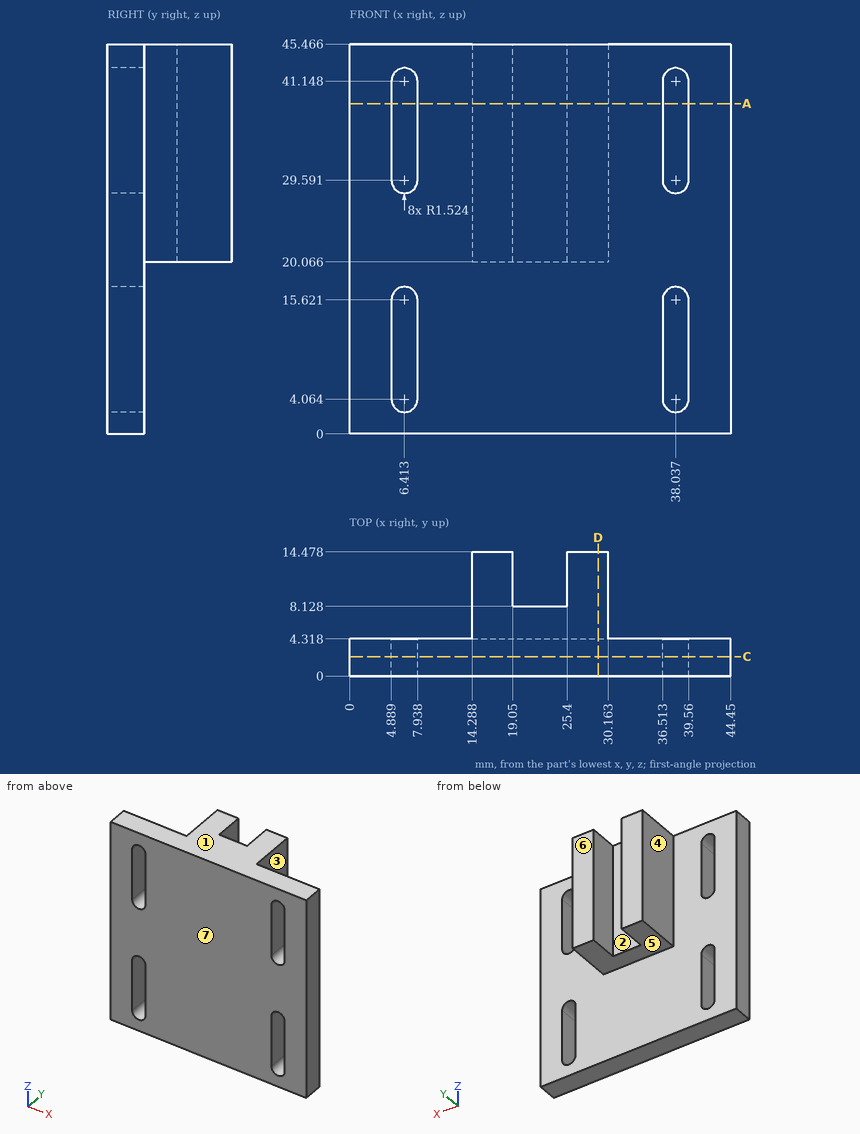
Source: three-view drawing plus pictorial views. Frame: mm from the lowest corner of the part. A direction names the side the tool comes from. Coordinates: 2 decimals unless noted, no trailing zeros. Order: outer loops, then holes, each group sorted by start corner. A loop starts at its lowest first (then second) coordinate and runs counter-clockwise, first axis right, second up. Notation, with made-up numbers: M -12.5,-32.5 L 17.5,-32.5 A10 ccw 17.5,-18.5 Z; hole C -11.5,76 d11. An arc over 180 degrees is marked long. One line per question, with ' | ' between items. Start each with the question number.
Item 1: Set-up query: the marked faces 1, 2, 3 and 4. Return all of +Z, -Z, +X, -X, +Y, -Y with unobstructed straight access to the full face (end or side cutting, diameter ignored); none if empty.
Item 2: Draft query along Y for the marked faces 5, 6 and 7. Return one class per face: released by +Y, released by -Y, zero draft, split by the parting line, or undercut.
Item 3: Ray query, probe 1 along X at (y, z) = (2.5, 13.5); probe 2 along X at (y, z) = (10.5, 38.5); probe 3 along Z at (x, y) = (7, 1) (1 decimal). Return the intervals inside material, ascending. Write a range as [from, to].
Item 4: Cut plane C-C, the plane y = 2.25. Count the separate pieces of the cut face and the enclosed holes in it, then the cut area to 3 significant figures.
Item 5: Pin query (flat end, axial travel): pin 1 Ø3 at (y, z) = (11, 32.5) entering from -X; pin 2 Ø5 at (x, y) = (38.5, 7) entering from +Z; pin 3 Ø5 at (x, y) = (21, 7.5) entering from -Z; pin 4 Ø10 at (x, z) = (5, 39) entering from +Y. Return the tip coordinate at first contact, or that it passes through.
Item 6: Cut plane A-A, the plane z = 38.5. Return the cut outline in (x, y).
Item 7: Cut plane D-D, the plane x = 29. Return the cut outline in (y, z) (1 decimal).
A:
1) face 1: +Z, +X, -X, +Y, -Y | face 2: +Z, -Z, +Y | face 3: +Z, -Z, +X, +Y | face 4: +Z, -Z, -X, +Y
2) face 5: zero draft | face 6: released by +Y | face 7: released by -Y
3) probe 1: x = [0, 4.89], [7.94, 36.51], [39.56, 44.45] | probe 2: x = [14.29, 19.05], [25.4, 30.16] | probe 3: z = [0, 2.7], [17, 28.2], [42.6, 45.5]
4) separate pieces: 1 | enclosed holes: 4 | area: 1,850 mm2
5) pin 1: stops at x = 14.29 | pin 2: passes through | pin 3: stops at z = 20.07 | pin 4: stops at y = 4.32
6) outline: M 0,0 L 4.89,0 L 4.89,4.32 L 0,4.32 Z; M 7.94,0 L 36.51,0 L 36.51,4.32 L 30.16,4.32 L 30.16,14.48 L 25.4,14.48 L 25.4,8.13 L 19.05,8.13 L 19.05,14.48 L 14.29,14.48 L 14.29,4.32 L 7.94,4.32 Z; M 39.56,0 L 44.45,0 L 44.45,4.32 L 39.56,4.32 Z
7) outline: M 0,0 L 4.3,0 L 4.3,20.1 L 14.5,20.1 L 14.5,45.5 L 0,45.5 Z
